from build123d import *

# Parameters (mm, degrees)
ESQUISSE1_W             = 8.928
ESQUISSE1_H             = 17.1
BOSS_EXTRU_1_DEPTH      = 1.227
ESQUISSE2_W             = 6.124
ESQUISSE2_H             = 11.244
BOSS_EXTRU_2_DEPTH      = 0.1
BOSS_EXTRU_4_DEPTH      = 8.928
ENL_V_MAT_EXTRU_1_REACH = 13.629
ESQUISSE5_W             = 1.364
ESQUISSE5_H             = 1


with BuildPart() as part:
    # Esquisse1 → Boss.-Extru.1 (new body)
    with BuildSketch(Plane.XY):
        Rectangle(ESQUISSE1_W, ESQUISSE1_H)
    extrude(amount=BOSS_EXTRU_1_DEPTH)

    # Esquisse2 → Boss.-Extru.2 (add)
    with BuildSketch(Plane.XY.offset(1.227)):
        with Locations((0, 1.525)):
            Rectangle(ESQUISSE2_W, ESQUISSE2_H)
    extrude(amount=BOSS_EXTRU_2_DEPTH)

    # Esquisse4 → Boss.-Extru.4 (add)
    with BuildSketch(Plane(origin=(4.464, 0, 0), x_dir=(0, 0, -1), z_dir=(1, 0, 0))):
        with BuildLine():
            Line((-1.227, -8.55), (-1.227, -9.55))
            ThreePointArc((-1.227, -9.55), (-0.227, -10.55), (0.773, -9.55))
            Line((0.773, -9.55), (0.773, -3.55))
            Line((0.773, -3.55), (0.673, -3.55))
            Line((0.673, -3.55), (0.673, -9.55))
            ThreePointArc((0.673, -9.55), (-0.227, -10.45), (-1.127, -9.55))
            Line((-1.127, -9.55), (-1.127, -8.55))
            Line((-1.127, -8.55), (-1.227, -8.55))
        make_face()
    extrude(amount=-BOSS_EXTRU_4_DEPTH)

    # Esquisse5 → Enlèv. mat.-Extru.1 (cut, up to next)
    with BuildSketch(Plane.XY.offset(1.227), mode=Mode.PRIVATE) as enl_v_mat_extru_1_sk1:
        with Locations((3.782, -10.05)):
            Rectangle(ESQUISSE5_W, ESQUISSE5_H)
    enl_v_mat_extru_1_tool1 = extrude(enl_v_mat_extru_1_sk1.sketch, amount=-ENL_V_MAT_EXTRU_1_REACH, mode=Mode.PRIVATE) & part.part
    # Esquisse5 → Enlèv. mat.-Extru.1 (cut, up to next)
    with BuildSketch(Plane.XY.offset(1.227), mode=Mode.PRIVATE) as enl_v_mat_extru_1_sk2:
        with Locations((-3.782, -10.05)):
            Rectangle(ESQUISSE5_W, ESQUISSE5_H)
    enl_v_mat_extru_1_tool2 = extrude(enl_v_mat_extru_1_sk2.sketch, amount=-ENL_V_MAT_EXTRU_1_REACH, mode=Mode.PRIVATE) & part.part
    add(enl_v_mat_extru_1_tool1.solids().sort_by_distance((3.782, -10.05, 1.227))[0], mode=Mode.SUBTRACT)
    add(enl_v_mat_extru_1_tool2.solids().sort_by_distance((-3.782, -10.05, 1.227))[0], mode=Mode.SUBTRACT)


solid = part.part
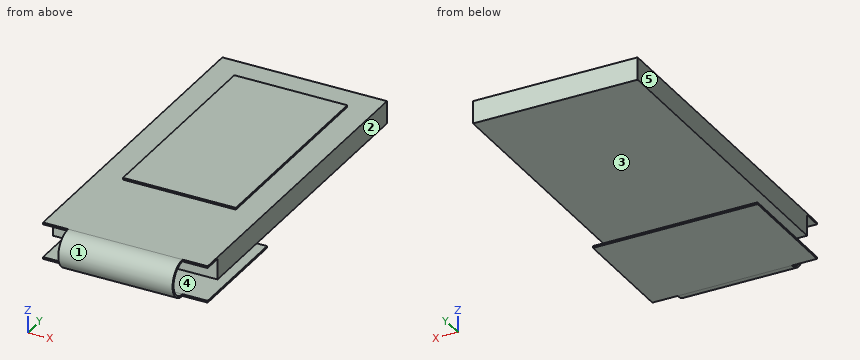
Geometry check sheet. Reference: the model listing, model coordinates, mm. Face numbers are marked on the shaded views. A direction names the side the tool comes from. Give positions to 0.01 mm unless a question says otherwise; leave off trailing zeros. Order: outer loops, then holes, each group sorted by start corner. A loop starts at its lowest first (then second) coordinate and runs counter-clockwise, first axis right, second up.
1) Cross-section at B-B (z = 0.55). Record the boundary of the cut face in (x, y).
Results are:
outline: (-4.46, -8.55) - (4.46, -8.55) - (4.46, 8.55) - (-4.46, 8.55) - close; (-3.1, -10.5) - (3.1, -10.5) - (3.1, -10.39) - (-3.1, -10.39) - close
2) Material ranges on probe 1 along Z at (x, y) = (4.25, 0.25); probe 2 along Z at (x, y) = (1.25, 2.25), recorded low to high.
Results are:
probe 1: z = 0 to 1.23
probe 2: z = 0 to 1.33
3) Tool access check on the marked faces 4 and 5. Record the directions out of +Z, -Z, +X, -X, +Y, -Y that give a thin tool (end or side, any length) a straight path to the whole face; none if there is none.
Results are:
face 4: +X, -X, +Y
face 5: +Z, -Z, -X, +Y, -Y
4) Cross-section at D-D (y = -0.75). Record the boundary of the cut face in (x, z), then the cut area to 3 significant figures.
Results are:
outline: (-4.46, 0) - (4.46, 0) - (4.46, 1.23) - (3.06, 1.23) - (3.06, 1.33) - (-3.06, 1.33) - (-3.06, 1.23) - (-4.46, 1.23) - close
area: 11.6 mm2
5) Draft check along Z on the marked faces 1, 2 and 3. Enter one of: released by +Z, released by -Z, zero draft, split by the parting line, or undercut.
Results are:
face 1: split by the parting line
face 2: zero draft
face 3: undercut
6) Gauge pin test, flat ends, axial feed: pin 1 (1.1 mm diameter, centred on y = -10, z = 0.5, fed in from +X); pin 2 (1.5 mm diameter, centred on x = -1, y = -8, fed in from +Z); pin 3 (3 mm diameter, centred on x = -2.5, y = 0, fed in from -Z). Record the tip position at first contact, or that the pin passes through.
Results are:
pin 1: stops at x = 3.1
pin 2: stops at z = 1.23
pin 3: stops at z = 0
7) Cross-section at C-C (x = 2.25). Record the boundary of the cut face in (y, z).
Results are:
outline: (-9.55, -0.77) - (-3.55, -0.77) - (-3.55, -0.67) - (-9.55, -0.67) arc R0.9 cw to (-9.55, 1.13) - (-8.55, 1.13) - (-8.55, 0) - (8.55, 0) - (8.55, 1.23) - (7.15, 1.23) - (7.15, 1.33) - (-4.1, 1.33) - (-4.1, 1.23) - (-9.55, 1.23) arc R1 ccw to start
8) Cross-section at A-A (y = -7.75). Record the boundary of the cut face in (x, z).
Results are:
outline: (-4.46, -0.77) - (4.46, -0.77) - (4.46, -0.67) - (-4.46, -0.67) - close; (-4.46, 0) - (4.46, 0) - (4.46, 1.23) - (-4.46, 1.23) - close
